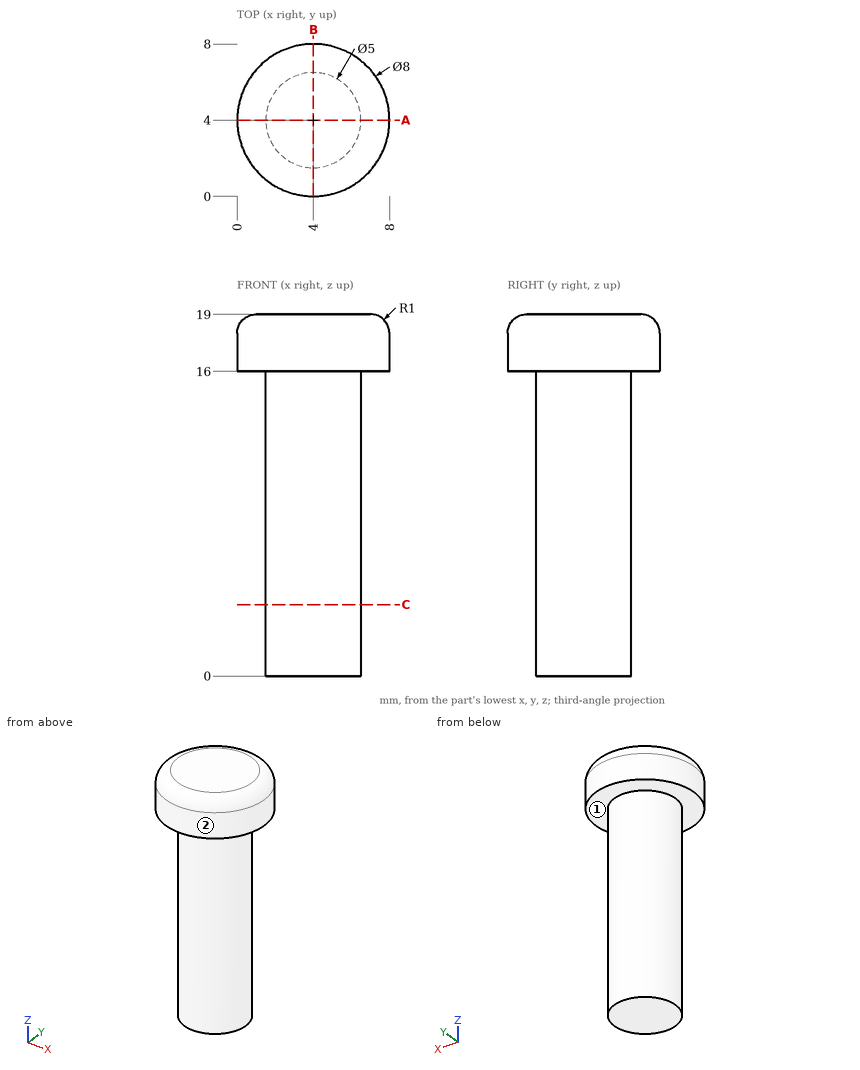
Input: dimensioned drawing with shaded views. Units: mm. Origin: part minimum x, y, z. A direction names the side the tool comes from. Coordinates: 2 decimals unless noted, no trailing zeros. Loops run counter-clockwise (first coordinate to the right, second up) from the corner with the lowest first, then second, coordinate; pieces in that order, holes last. Notation, with made-up numbers: M -13,10 L -5,10 A37 cw -5,47 Z; hole C 79.25,65 d9. An arc over 180 degrees is marked long. One line per item, written item: value. Start each with the question number.
1) Cut plane A-A (y = 4). Return loops of the section in (x, z).
2) Reachability of the marked faces 1 and 2 from +Z, -Z, +X, -X, +Y, -Y: full face, straight path, thin tool, end or side. Return the list, or none.
3) Cut plane C-C (z = 3.75). Return loops of the section in (x, y), then the cut area to 3 significant figures.
4) Material intervals for L1, parallel to Z at x = 1.5, y = 3.5; L2, parallel to X at y = 6.25, z = 11; L3, parallel to X at y = 2.25, z = 9.5, sorted ascending. Write a range as from..to.
5) Pin query (flat end, axial travel): P1, Ø1.5, axis at x = 6, z = 12, coming from the -Y side; P2, Ø1, axis at y = 3.5, z = 12.5, coming from the +X side; P3, Ø1.5, axis at y = 4.5, z = 11.5, coming from the -X side. Return the tip coordinate at first contact, or that it passes through.
Evaluation:
1. outline: M 0,16 L 1.5,16 L 1.5,0 L 6.5,0 L 6.5,16 L 8,16 L 8,18 A1 ccw 7,19 L 1,19 A1 ccw 0,18 Z
2. face 1: -Z
2. face 2: +Z, -Z
3. outline: C 4,4 d5
3. area: 19.6 mm^2
4. L1: 16..19
4. L2: 2.91..5.09
4. L3: 2.21..5.79
5. P1: y = 1.83
5. P2: x = 6.5
5. P3: x = 1.5
